from build123d import *

# Parameters (mm, degrees)
F1_DEPTH = 4.5
F1_TAPER = -3
F2_R     = 2.5
F3_DEPTH = 25
F4_SIZE  = 0.3


with BuildPart() as f1:
    # F0 (on Top) → F1 (new body)
    with BuildSketch(Plane.XY):
        Polygon((-1.2996787849, -4), (1.2996787849, -4), (3.4026032334, -2.472135955), (4.205848897, 0), (3.4026032334, 2.472135955), (1.2996787849, 4), (-1.2996787849, 4), (-3.4026032334, 2.472135955), (-4.205848897, 0), (-3.4026032334, -2.472135955), align=None)
    extrude(amount=F1_DEPTH, taper=F1_TAPER)

    # F2 (on face) → F3 (cut)
    with BuildSketch(Plane(origin=(0, 0, 0), x_dir=(1, 0, 0), z_dir=(0, 0, -1))):
        Circle(F2_R)
    extrude(amount=-F3_DEPTH, mode=Mode.SUBTRACT)

    # F4
    f4_edges = [f1.edges().sort_by_distance(p)[0] for p in [
        (-2.5, 0, 0),
        (-2.5, 0, 4.5),
    ]]
    chamfer(f4_edges, length=F4_SIZE)


solid = f1.part
Verification items for the finished model (mm, model axes). Coordinates: 2 decimals unless noted, no trailing zeros. One line per item, written item: value. Start each with the question number.
Item 1: Depth check by flat-ended pin: P1, Ø1, axis at x = -1, y = -2, coming from the +Z side; P2, Ø4, axis at x = -3, y = 1, coming from the -Z side. Enter the tip coordinate at first touch or a pass-through.
Item 2: Thickness scan on probe 1 along X at (y, z) = (0.25, 0.35); probe 2 along Y at (x, z) = (0, 1.65); probe 3 along X at (y, z) = (-2, 2.25). Record the ranges inside material, lowest first.
Item 3: Mould release check, pull along X, two halves, no side actions. Record for faces 1 (the flat face through (-1, -3, 0)), 2 (the cylindrical face through (-0.54, 2.44, 2.22)): pulls with the +X half, pulls with the -X half, needs draft (parallel to the pull), parting line crosses it, or undercut.
Calculated:
1. P1: z = 4.44
1. P2: z = 0
2. probe 1: -4.14 to -2.49, 2.49 to 4.14
2. probe 2: -4.09 to -2.5, 2.5 to 4.09
2. probe 3: -3.68 to -1.5, 1.5 to 3.68
3. face 1: needs draft
3. face 2: undercut
